Verification items for the finished model (mm, model axes). A direction names the side the tool comes from. Coordinates: 2 decimals unless noted, no trailing zeros. Loops run counter-clockwise (first coordinate to the right, second up) from the corner with the lowest first, then second, coordinate; pieces in that order, holes last. Notation, with made-up numbers: (2, -28.75) -> (31, -28.75) arc R38 ccw to (31, 9.25) -> close; hole circle Ø6 at (46, -10). An arc over 180 degrees is marked (long way). Write item = value, one per line.
```python
from build123d import *

# Parameters (mm, degrees)
ESQUISSE3_W                  = 6.57785754
ESQUISSE3_H                  = 1.386048805
ENL_V_MAT_EXTRU_1_DEPTH      = 28.5
D_GAGEMENT_M21_D             = 2.4
R_P_TITION_CIRCULAIRE1_COUNT = 4
CONG_1_R                     = 0.05


with BuildPart() as part:
    # Esquisse2 → Révolution2 (revolve)
    with BuildSketch(Plane.XY, mode=Mode.PRIVATE) as r_volution2_sk:
        Polygon((0, 35), (3.15, 35), (3.15, 6.5), (6.2, 6.5), (6.2, 3), (6.2, 1), (10, 1), (10, 0), (4.5, 0), (4.5, 3), (0, 3), align=None)
    revolve(r_volution2_sk.sketch.rotate(Axis((0, 3, 0), (0, 1, 0)), 90), axis=Axis((0, 3, 0), (0, 1, 0)))

    # Esquisse3 → Enlèv. mat.-Extru.1 (cut)
    with BuildSketch(Plane(origin=(0, 35, 0), x_dir=(1, 0, 0), z_dir=(0, 1, 0))):
        with Locations((-0.352413472, 3.114928535)):
            Rectangle(ESQUISSE3_W, ESQUISSE3_H)
    extrude(amount=-ENL_V_MAT_EXTRU_1_DEPTH, mode=Mode.SUBTRACT)

    # Dégagement M21 (through all)
    with Locations(Plane(origin=(0, 1, 0), x_dir=(1, 0, 0), z_dir=(0, 1, 0))):
        with Locations((0.371303159, 7.991378727)):
            d_gagement_m21 = Hole(D_GAGEMENT_M21_D / 2)

    # Répétition circulaire1: Dégagement M21 ×4 about axis
    r_p_tition_circulaire1_axis = Axis((0, 0, 0), (0, 1, 0))
    for i in range(1, R_P_TITION_CIRCULAIRE1_COUNT):
        add(d_gagement_m21.rotate(r_p_tition_circulaire1_axis, i * 360 / R_P_TITION_CIRCULAIRE1_COUNT), mode=Mode.SUBTRACT)

    # Congé1
    cong_1_edges = [part.edges().sort_by_distance(p)[0] for p in [
        (0, 6.5, 6.2),
        (0, 6.5, 3.15),
        (0, 35, 3.15),
        (0, 1, 6.2),
    ]]
    fillet(cong_1_edges, radius=CONG_1_R)


solid = part.part
```
1) Release check for a two-part mould opening along X. For faces 1 (the face through (-1.9, 3.8, -5.9)), 2 (the face through (-6.82, 0.49, -0.63)), 3 (the face through (0, 35, 0)) record: pulls with the +X half, pulls with the -X half, needs draft (parallel to the pull), parting line crosses it, or undercut.
Ans:
face_1 = parting line crosses it
face_2 = undercut
face_3 = needs draft
2) Sectioned sample at D-D, the plane y = 16. Record the cut outline in (x, z).
Ans:
outline = (-2.01, -2.42) -> (2.01, -2.42) arc R3.15 ccw (long way) to start
3) Sectioned sample at B-B, the plane y = 2. Record the cut outline in (x, z), plus the area to 3 significant figures.
Ans:
outline = circle Ø12.4 at (0, 0); hole circle Ø9 at (0, 0)
area = 57.1 mm2
4) Sectioned sample at A-A, the plane x = 0. Count the separate pieces of the cut face and the enclosed holes in it, plus the area to 3 significant figures.
Ans:
separate_pieces = 3
enclosed_holes = 0
area = 215 mm2
5) Depth check by flat-ended pin: pin 1 Ø1.5 at (x, z) = (0, 1) entering from -Y; pin 2 Ø4 at (x, z) = (7.99, 0.37) entering from +Y; pin 3 Ø4.5 at (x, y) = (-0.5, 16) entering from -Z. Enter the tip coordinate at first touch or a pass-through.
Ans:
pin_1 = 3
pin_2 = 6.5
pin_3 = -2.42
6) Material ranges on line 1 (X direction, y = 2, z = 0); line 2 (Y direction, x = 3.5, z = 5.25); line 3 (Y direction, x = 4.75, z = 2), recorded low to high.
Ans:
line_1 = -6.2 to -4.5, 4.5 to 6.2
line_2 = 0 to 1
line_3 = 0 to 6.5
7) Tool access check on faces 4 (the face through (0, 21, -2.422)), 5 (the face through (0, 3, 0)), 6 (the face through (-5, 1, 4)), 7 (the face through (4.3, 0, -2.1)), 8 (the face through (-0.63, 0.49, 6.82)). Record the directions out of +Z, -Z, +X, -X, +Y, -Y that give a thin tool (end or side, any length) a straight path to the whole face; none if there is none.
Ans:
face_4 = -Z, +X, -X, +Y
face_5 = -Y
face_6 = +Y
face_7 = +Z, -Z, +X, -X, -Y
face_8 = +Y, -Y
